from build123d import *

# Parameters (mm, degrees)
CUT_EXTRUDE1_REACH = 13


with BuildPart() as part:
    # Sketch2 → Revolve1 (revolve)
    with BuildSketch(Plane.XY):
        Polygon((-25, 2.5), (-25, -2.5), (-30, -2.5), (-30, -5.5), (0, -5.5), (0, 5.5), (-30, 5.5), (-30, 2.5), align=None)
    revolve(axis=Axis((0, 19.987411147, 0), (0, -1, 0)))

    # Sketch3 → Cut-Extrude1 (cut, up to next)
    with BuildSketch(Plane(origin=(0, 5.5, 0), x_dir=(1, 0, 0), z_dir=(0, 1, 0)), mode=Mode.PRIVATE) as cut_extrude1_sk1:
        with BuildLine():
            ThreePointArc((15.055438643, -16.720758573), (19.485571585, -11.25), (22.008321017, -4.678013043))
            Line((22.008321017, -4.678013043), (15.161287811, -3.222631208))
            ThreePointArc((15.161287811, -3.222631208), (15.367467985, -2.022604196), (15.478816003, -0.810095759))
            Line((15.478816003, -0.810095759), (22.395997522, 2.160855156))
            ThreePointArc((22.395997522, 2.160855156), (19.485571585, 11.25), (13.06935422, 18.315075219))
            Line((13.06935422, 18.315075219), (7.037844495, 13.810095759))
            ThreePointArc((7.037844495, 13.810095759), (5.932107377, 14.319919765), (4.789763413, 14.741376003))
            Line((4.789763413, 14.741376003), (6.952882373, 21.398771617))
            ThreePointArc((6.952882373, 21.398771617), (0, 22.5), (-6.952882373, 21.398771617))
            Line((-6.952882373, 21.398771617), (-4.789763413, 14.741376003))
            ThreePointArc((-4.789763413, 14.741376003), (-5.932107377, 14.319919765), (-7.037844495, 13.810095759))
            Line((-7.037844495, 13.810095759), (-13.06935422, 18.315075219))
            ThreePointArc((-13.06935422, 18.315075219), (-19.485571585, 11.25), (-22.395997522, 2.160855156))
            Line((-22.395997522, 2.160855156), (-15.478816003, -0.810095759))
            ThreePointArc((-15.478816003, -0.810095759), (-15.367467985, -2.022604196), (-15.161287811, -3.222631208))
            Line((-15.161287811, -3.222631208), (-22.008321017, -4.678013043))
            ThreePointArc((-22.008321017, -4.678013043), (-19.485571585, -11.25), (-15.055438643, -16.720758573))
            Line((-15.055438643, -16.720758573), (-10.371524399, -11.518744795))
            ThreePointArc((-10.371524399, -11.518744795), (-9.435360608, -12.297315569), (-8.440971508, -13))
            Line((-8.440971508, -13), (-9.326643302, -20.475930375))
            ThreePointArc((-9.326643302, -20.475930375), (0, -22.5), (9.326643302, -20.475930375))
            Line((9.326643302, -20.475930375), (8.440971508, -13))
            ThreePointArc((8.440971508, -13), (9.435360608, -12.297315569), (10.371524399, -11.518744795))
            Line((10.371524399, -11.518744795), (15.055438643, -16.720758573))
        make_face()
    cut_extrude1_tool1 = extrude(cut_extrude1_sk1.sketch, amount=-CUT_EXTRUDE1_REACH, mode=Mode.PRIVATE) & part.part
    add(cut_extrude1_tool1.solids().sort_by_distance((0, 5.5, 0))[0], mode=Mode.SUBTRACT)


solid = part.part
Could you check a few things on this model? Use its own coordinates, in mm. Give positions to 0.01 mm unless a question says otherwise; leave off trailing zeros. Order: outer loops, then holes, each group sorted by start corner. A loop starts at its lowest first (then second) coordinate and runs counter-clockwise, first axis right, second up. Notation, with made-up numbers: (16.25, -19.75) - (46.25, -19.75) arc R18 cw to (46.25, 12.25) - close; hole circle Ø7 at (89.25, 30.25). An arc over 180 degrees is marked (long way). Return JSON: item names as keys, results as strings. Group by question number.
Q1. Please list where these lines run through material, in increasing order: line 1 along Y through (x, z) = (27, -1); line 2 along X through (y, z) = (0, -8.5); line 3 along X through (y, z) = (3.25, 18.5). Write a range as [from, to].
Q2. Thinking about a two-plate mould opening in Y: for faces 1 (the face through (-23.846, -0.035, -7.509)), 2 (the face through (-12.75, 0.08, 14.16)), 3 (the face through (20, 5.5, 0)), which applies, pulls with the +Y half, pulls with the -Y half, needs draft (parallel to the pull), parting line crosses it, or undercut?
Q3. Will these pins go through, and if not, where does the flat tip stop? pin 1 Ø4 at (x, y) = (4.5, 4) entering from -Z; pin 2 Ø2 at (x, y) = (-20, -3.5) entering from +Z.
Q4. Suppose I cut it at B-B, the plane y = 1.5. Please give me the cut outline in (x, z).
Q5. Suppose I cut it at A-A, the plane x = 0. Please give me the cut outline in (y, z), and give its area (3 significant figures).
Q6. Suppose I cut it at D-D, the plane y = -4.25. Please give me the cut outline in (x, z), and give its area (3 significant figures).
Q7. Suppose I cut it at C-C, the plane z = 0. Please give me the cut outline in (x, y), and give its area (3 significant figures).
Resolved:
{
 "1": {"line 1": "y = [-5.5, -2.5], [2.5, 5.5]", "line 2": "x = [-23.51, -20.83], [20.83, 23.51]", "line 3": "x = [-23.62, -9.09], [9.09, 23.62]"},
 "2": {"face 1": "undercut", "face 2": "needs draft", "face 3": "pulls with the +Y half"},
 "3": {"pin 1": "stops at z = -29.9", "pin 2": "stops at z = 23.22"},
 "4": {"outline": "circle Ø50 at (0, 0); hole (-22.4, -2.16) arc R22.5 ccw to (-13.07, -18.32) - (-7.04, -13.81) arc R15.5 ccw to (-4.79, -14.74) - (-6.95, -21.4) arc R22.5 ccw to (6.95, -21.4) - (4.79, -14.74) arc R15.5 ccw to (7.04, -13.81) - (13.07, -18.32) arc R22.5 ccw to (22.4, -2.16) - (15.48, 0.81) arc R15.5 ccw to (15.16, 3.22) - (22.01, 4.68) arc R22.5 ccw to (15.06, 16.72) - (10.37, 11.52) arc R15.5 ccw to (8.44, 13) - (9.33, 20.48) arc R22.5 ccw to (-9.33, 20.48) - (-8.44, 13) arc R15.5 ccw to (-10.37, 11.52) - (-15.06, 16.72) arc R22.5 ccw to (-22.01, 4.68) - (-15.16, 3.22) arc R15.5 ccw to (-15.48, 0.81) - close"},
 "5": {"outline": "(-5.5, -30) - (-2.5, -30) - (-2.5, -25) - (2.5, -25) - (2.5, -30) - (5.5, -30) - (5.5, -22.5) - (-5.5, -22.5) - close; (-5.5, 22.5) - (5.5, 22.5) - (5.5, 30) - (2.5, 30) - (2.5, 25) - (-2.5, 25) - (-2.5, 30) - (-5.5, 30) - close", "area": "115 mm2"},
 "6": {"outline": "circle Ø60 at (0, 0); hole (-22.4, -2.16) arc R22.5 ccw to (-13.07, -18.32) - (-7.04, -13.81) arc R15.5 ccw to (-4.79, -14.74) - (-6.95, -21.4) arc R22.5 ccw to (6.95, -21.4) - (4.79, -14.74) arc R15.5 ccw to (7.04, -13.81) - (13.07, -18.32) arc R22.5 ccw to (22.4, -2.16) - (15.48, 0.81) arc R15.5 ccw to (15.16, 3.22) - (22.01, 4.68) arc R22.5 ccw to (15.06, 16.72) - (10.37, 11.52) arc R15.5 ccw to (8.44, 13) - (9.33, 20.48) arc R22.5 ccw to (-9.33, 20.48) - (-8.44, 13) arc R15.5 ccw to (-10.37, 11.52) - (-15.06, 16.72) arc R22.5 ccw to (-22.01, 4.68) - (-15.16, 3.22) arc R15.5 ccw to (-15.48, 0.81) - close", "area": "1,430 mm2"},
 "7": {"outline": "(-30, -5.5) - (-17.36, -5.5) - (-17.36, 5.5) - (-30, 5.5) - (-30, 2.5) - (-25, 2.5) - (-25, -2.5) - (-30, -2.5) - close; (17.36, -5.5) - (30, -5.5) - (30, -2.5) - (25, -2.5) - (25, 2.5) - (30, 2.5) - (30, 5.5) - (17.36, 5.5) - close", "area": "228 mm2"}
}
